Autodesk Inventor part; units mm, degrees
ref_plane "YZ Plane" through (0, 0, 0) normal (1, 0, 0) x (0, 1, 0)
ref_plane "XZ Plane" through (0, 0, 0) normal (0, 1, 0) x (-1, 0, 0)
ref_plane "XY Plane" through (0, 0, 0) normal (0, 0, 1) x (1, 0, 0)
sketch "Szkic1" plane through (0, 0, 0) normal (0, 0, 1) x (1, 0, 0)
  line L0 (0, 0) -> (20, 0)
  line L1 (0, 0) -> (-20, 0)
  line L2 (-20, 0) -> (-20, 20)
  line L3 (-20, 0) -> (0, 0) construction
  line L4 (-20, 20) -> (20, 20)
  line L5 (20, 20) -> (20, 0)
  line L6 (-20, 0) -> (-20, 88)
  line L7 (-20, 88) -> (20, 88)
  line L8 (20, 88) -> (20, 20)
  line L9 (20, 88) -> (20, 93)
  line L10 (20, 93) -> (-20, 93)
  line L11 (-20, 93) -> (-20, 88)
  line L12 (0, 93) -> (35, 93)
  line L13 (35, 93) -> (40, 93)
  line L14 (0, 93) -> (-35, 93)
  line L15 (-35, 93) -> (-40, 93)
  line L16 (-40, 93) -> (-40, 103)
  line L17 (-40, 103) -> (40, 103)
  line L18 (40, 103) -> (40, 93)
  line L19 (-35, 93) -> (-35, 103)
  line L20 (35, 93) -> (35, 103)
  circle A0 centre (-35, 103) radius 1.5
  circle A1 centre (-35, 93) radius 1.5
  circle A2 centre (35, 103) radius 1.5
  circle A3 centre (35, 93) radius 1.5
  line L21 (40, 93) -> (40, 83)
  line L22 (40, 83) -> (20, 83)
  line L23 (-40, 93) -> (-40, 83)
  line L24 (-40, 83) -> (-20, 83)
  line L25 (-40, 103) -> (-40, 183)
  line L26 (40, 103) -> (40, 183)
  line L27 (40, 183) -> (-40, 183)
  dimension "d0" = 20
  dimension "d1" = 20
  dimension "d2" = 20
  dimension "d3" = 90
  dimension "d4" = 88
  dimension "d5" = 5
  dimension "d6" = 35
  dimension "d7" = 5
  dimension "d8" = 35
  dimension "d9" = 5
  dimension "d10" = 10
  dimension "d11" = 3
  dimension "d12" = 3
  dimension "d13" = 3
  dimension "d14" = 3
  dimension "d15" = 10
  dimension "d16" = 10
  dimension "d17" = 80
  dimension "d18" = 80
extrude "Wyciągnięcie proste1" add sketch "Szkic1" along normal blind 8
sketch "Szkic2" plane through (0, 0, 8) normal (0, 0, 1) x (1, 0, 0)
  circle A0 centre (-35, 103) radius 1.5
  circle A1 centre (-35, 93) radius 1.5
  circle A2 centre (35, 103) radius 1.5
  circle A3 centre (35, 93) radius 1.5
  line L0 (-35, 103) -> (35, 103)
  line L1 (-35, 93) -> (35, 93)
  line L2 (-35, 103) -> (-20, 103)
  line L3 (-20, 103) -> (-20, 93)
  line L4 (35, 103) -> (20, 103)
  line L5 (20, 103) -> (20, 93)
  circle A4 centre (-20, 103) radius 2
  circle A5 centre (-20, 93) radius 2
  circle A6 centre (20, 103) radius 2
  circle A7 centre (20, 93) radius 2
  line L6 (40, 83) -> (40, 183)
  line L7 (40, 183) -> (-40, 183)
  line L8 (-40, 183) -> (-40, 83)
  line L9 (-40, 83) -> (-20, 83)
  line L10 (-20, 83) -> (-20, 0)
  line L11 (-20, 0) -> (20, 0)
  line L12 (20, 0) -> (20, 83)
  line L13 (20, 83) -> (40, 83)
  line L14 (-20, 0) -> (20, 0)
  line L15 (-20, 0) -> (-20, 10)
  line L16 (-20, 83) -> (-20, 0)
  line L17 (-20, 10) -> (20, 10)
  line L18 (-20, 10) -> (-10, 10)
  line L19 (20, 10) -> (10, 10)
  circle A8 centre (-10, 10) radius 3
  circle A9 centre (10, 10) radius 3
  point P0 (0, 0)
  dimension "d21" = 15
  dimension "d22" = 15
  dimension "d23" = 4
  dimension "d24" = 4
  dimension "d25" = 4
  dimension "d26" = 4
  dimension "d27" = 10
  dimension "d28" = 10
  dimension "d29" = 10
  dimension "d30" = 6
  dimension "d31" = 6
hole "Otwór1" at (-20, 103, 8) at (-20, 93, 8) at (20, 103, 8) at (20, 93, 8) at (-35, 103, 8) at (-35, 93, 8) at (35, 103, 8) at (35, 93, 8) direction (0, 0, -1) diameter 4 end through all
sketch "Szkic3" plane through (0, 0, 8) normal (0, 0, 1) x (1, 0, 0)
  circle A0 centre (-10, 10) radius 3
  circle A1 centre (10, 10) radius 3
  point P0 (0, 0)
hole "Otwór2" at (-10, 10, 8) at (10, 10, 8) direction (0, 0, -1) diameter 6 end through all
fillet "Zaokrąglenie1" radius 20 2 edges at (20, 83, 4) (-20, 83, 4)
sketch "Szkic4" plane through (0, 0, 8) normal (0, 0, 1) x (1, 0, 0)
  line L0 (40, 183) -> (-40, 183)
  line L1 (40, 83) -> (40, 183)
  line L2 (40, 183) -> (-40, 183)
  line L3 (-40, 183) -> (-40, 333)
  line L4 (-40, 333) -> (0, 333)
  line L5 (40, 183) -> (40, 233)
  line L6 (40, 233) -> (0, 333)
  point P0 (0, 0)
  dimension "d47" = 150
  dimension "d50" = 50
extrude "Wyciągnięcie proste2" add sketch "Szkic4" against normal up to surface (8 mm away)
sketch "Szkic5" plane through (0, 0, 8) normal (0, 0, 1) x (1, 0, 0)
  line L0 (0, 333) -> (-40, 333)
  line L1 (-40, 333) -> (-40, 83)
  line L2 (-40, 333) -> (-40, 308)
  line L3 (-40, 308) -> (-17, 308)
  circle A0 centre (-17, 308) radius 15
  point P0 (0, 0)
  dimension "d51" = 25
  dimension "d52" = 23
  dimension "d53" = 30
extrude "Wyciągnięcie proste3" cut sketch "Szkic5" against normal up to next
sketch "Szkic6" plane through (0, 0, 8) normal (0, 0, 1) x (1, 0, 0)
  line L0 (40, 233) -> (0, 333)
  line L1 (0, 333) -> (10, 333)
  line L2 (10, 333) -> (40, 233)
  point P0 (0, 0)
  dimension "d56" = 10
extrude "Wyciągnięcie proste4" add sketch "Szkic6" against normal blind 8
sketch "Szkic7" plane through (0, 0, 0) normal (0, 0, -1) x (-1, 0, 0)
  line L0 (40, 83) -> (40, 333)
  line L1 (40, 333) -> (40, 263)
  line L2 (40, 263) -> (0, 263)
  line L3 (0, 263) -> (0, 183)
  line L4 (0, 183) -> (40, 183)
  line L5 (40, 263) -> (20, 263)
  line L6 (20, 263) -> (20, 183)
  line L7 (20, 263) -> (20, 253)
  line L8 (20, 183) -> (20, 213)
  circle A0 centre (20, 253) radius 4.5
  circle A1 centre (20, 213) radius 4.5
  point P0 (0, 0)
  dimension "d59" = 70
  dimension "d60" = 40
  dimension "d61" = 80
  dimension "d62" = 20
  dimension "d63" = 10
  dimension "d64" = 30
  dimension "d65" = 9
  dimension "d66" = 9
extrude "Wyciągnięcie proste5" cut sketch "Szkic7" against normal up to next contours A1 L6 | L6 A1 | A0 L6 | L6 A0
properties part number "Wspornik pionowy osi Y - lewa strona"
Geometry check sheet. Reference: the model listing, model coordinates, mm. A direction names the side the tool comes from. Coordinates: 2 decimals unless noted, no trailing zeros. Order: outer loops, then holes, each group sorted by start corner. A loop starts at its lowest first (then second) coordinate and runs counter-clockwise, first axis right, second up. Notation, with made-up numbers: (88, 39) - (108, 39) arc R29 cw to (108, 63) - close; hole circle Ø3 at (14, -32). An arc over 180 degrees is marked (long way). Answer in a Markdown table with one row per item. Add a question column.
1. Section check D-D (y = 213). Enter the section's corners in (x, z), plus the area to 3 significant figures.
2. Gauge pin test, flat ends, axial feed: pin 1 Ø14.5 at (x, y) = (-20, 253) entering from -Z; pin 2 Ø2 at (y, z) = (57, 1.5) entering from +X; pin 3 Ø3.5 at (x, y) = (20, 93) entering from -Z; pin 4 Ø4 at (y, z) = (32, 3) entering from -X. Record the tip position at first contact, or that the pin passes through.
3. Material ranges on L1, parallel to X at y = 103, z = 2.25; L2, parallel to X at y = 213, z = 3.75; L3, parallel to Y at x = -10, z = 6.25, recorded low to high. Write a range as [from, to].
4. Section check A-A (y = 253). Enter the section's corners in (x, z).
5. Draft check along X on faces 3 (the face through (20, 32, 4)), 4 (the face through (-15, 333, 4)), 5 (the face through (7.97, 12.21, 3.94)). Enter one of: +X half, -X half, draft (parallel to the pull), parting line (faces both ways), or undercut.
6. Section check C-C (z = 4). Give the number of separate pieces and of enclosed holes in the cut face, plus the area to 3 significant figures.
7. Access from +Z, -Z, +X, -X, +Y, -Y to the whole of each face (thin tool, end or side, straight path). Record for faces 1 (the face through (-19.02, 248.61, 3.94)), 2 (the face through (-20, 31, 4)).
8. Section check B-B (x = -10). Enter the section's corners in (y, z), plus the area to 3 significant figures.
Data:
| question | item | result |
|---|---|---|
| 1 | outline | (-40, 0) - (-24.5, 0) - (-24.5, 8) - (-40, 8) - close; (-15.5, 0) - (40, 0) - (40, 8) - (-15.5, 8) - close |
| 1 | area | 568 mm² |
| 2 | pin 1 | stops at z = 0 |
| 2 | pin 2 | stops at x = 20 |
| 2 | pin 3 | passes through |
| 2 | pin 4 | stops at x = -20 |
| 3 | L1 | x = [-40, -37], [-33, -22], [-18, 18], [22, 33], [37, 40] |
| 3 | L2 | x = [-40, -24.5], [-15.5, 40] |
| 3 | L3 | y = [0, 7], [13, 294.73], [321.27, 333] |
| 4 | outline | (-40, 0) - (-24.5, 0) - (-24.5, 8) - (-40, 8) - close; (-15.5, 0) - (34, 0) - (34, 8) - (-15.5, 8) - close |
| 5 | face 3 | +X half |
| 5 | face 4 | draft |
| 5 | face 5 | undercut |
| 6 | separate pieces | 1 |
| 6 | enclosed holes | 13 |
| 6 | area | 21,000 mm² |
| 7 | face 1 | +Z, -Z |
| 7 | face 2 | +Z, -Z, -X, -Y |
| 8 | outline | (0, 0) - (7, 0) - (7, 8) - (0, 8) - close; (13, 0) - (294.73, 0) - (294.73, 8) - (13, 8) - close; (321.27, 0) - (333, 0) - (333, 8) - (321.27, 8) - close |
| 8 | area | 2,400 mm² |
